from build123d import *

# Parameters (mm, degrees)
BOSS_EXTRUDE1_DEPTH  = 10
MIRROR1_DEPTH        = 10
SKETCH2_R            = 17.5
SKETCH2_R_2          = 15.5
BOSS_EXTRUDE2_DEPTH  = 5
CUT_EXTRUDE2_START   = -5
SKETCH3_R            = 15.5
CUT_EXTRUDE2_DEPTH   = 5
SKETCH4_R            = 12.5
CUT_EXTRUDE3_DEPTH   = 81.734131568
CHAMFER2_SIZE        = 0.2
CHAMFER4_SIZE        = 0.5
SKETCH5_R            = 5
SKETCH5_R_2          = 21
CUT_EXTRUDE5_DEPTH   = 1
CHAMFER6_SIZE        = 1
SKETCH6_R            = 0.75
CUT_EXTRUDE6_DEPTH   = 7
SKETCH7_R            = 0.75
CUT_EXTRUDE7_DEPTH   = 7
CUT_EXTRUDE8_DEPTH   = 151.432709209
CUT_EXTRUDE9_DEPTH   = 100.548982918
CUT_EXTRUDE10_DEPTH  = 81.616375508
FILLET3_R            = 2
FILLET3_OF_MIRROR3_R = 2
SKETCH11_R           = 0.75
CUT_EXTRUDE11_DEPTH  = 5


# Read off the part's stored shape, not the designer's step: Mirror1
with BuildPart() as part:
    # Sketch1 → Boss-Extrude1 (new body)
    with BuildSketch(Plane(origin=(0, 0, 0), x_dir=(1, 0, 0), z_dir=(0, 1, 0))):
        Polygon((-73, 31), (-71, 33), (-63, 33), (-61, 31), (-7, 31), (-5, 33), (0, 33), (0, 0), (-73, 0), (-73, 5), (-71, 7), (-71, 21), (-73, 23), align=None)
    extrude(amount=BOSS_EXTRUDE1_DEPTH)

    # Mirror1 outline → Mirror1 (add)
    with BuildSketch(Plane(origin=(0, 0, 0), x_dir=(1, 0, 0), z_dir=(0, 1, 0))):
        Polygon((-73, 0), (-73, -5), (-71, -7), (-71, -21), (-73, -23), (-73, -31), (-71, -33), (-63, -33), (-61, -31), (-7, -31), (-5, -33), (5, -33), (7, -31), (61, -31), (63, -33), (71, -33), (73, -31), (73, -23), (71, -21), (71, -7), (73, -5), (73, 5), (71, 7), (71, 21), (73, 23), (73, 31), (71, 33), (63, 33), (61, 31), (7, 31), (5, 33), (0, 33), (0, 0), align=None)
    extrude(amount=MIRROR1_DEPTH)

    # Sketch2 → Boss-Extrude2 (add)
    with BuildSketch(Plane(origin=(0, 10, 0), x_dir=(1, 0, 0), z_dir=(0, 1, 0))):
        with Locations(Location((0, 0, 0), (0, 0, 90))):
            Circle(SKETCH2_R)
        with Locations(Location((0, 0, 0), (0, 0, 270))):
            Circle(SKETCH2_R_2, mode=Mode.SUBTRACT)
    extrude(amount=BOSS_EXTRUDE2_DEPTH)

    # Sketch3 → Cut-Extrude2 (cut)
    with BuildSketch(Plane(origin=(0, 10, 0), x_dir=(1, 0, 0), z_dir=(0, 1, 0)).offset(CUT_EXTRUDE2_START)):
        with Locations(Location((0, 0, 0), (0, 0, 270))):
            Circle(SKETCH3_R)
    extrude(amount=CUT_EXTRUDE2_DEPTH, mode=Mode.SUBTRACT)

    # Sketch4 → Cut-Extrude3 (cut, through all)
    with BuildSketch(Plane(origin=(0, 5, 0), x_dir=(1, 0, 0), z_dir=(0, 1, 0))):
        with Locations(Location((0, 0, 0), (0, 0, 270))):
            Circle(SKETCH4_R)
    extrude(amount=-CUT_EXTRUDE3_DEPTH, mode=Mode.SUBTRACT)

    # Chamfer2
    chamfer2_edges = [part.edges().sort_by_distance(p)[0] for p in [
        (0, 15, 17.5),
        (0, 15, -15.5),
    ]]
    chamfer(chamfer2_edges, length=CHAMFER2_SIZE)

    # Chamfer4
    chamfer4_edges = [part.edges().sort_by_distance(p)[0] for p in [
        (0, 0, -12.5),
        (0, 5, -12.5),
    ]]
    chamfer(chamfer4_edges, length=CHAMFER4_SIZE)

    # Sketch5 → Cut-Extrude5 (cut)
    with BuildSketch(Plane.XZ.offset(-10)):
        Polygon((71, 4.171572875), (69, 6.171572875), (69, 21.828427125), (71, 23.828427125), (71, 30.171572875), (70.171572875, 31), (63.828427125, 31), (61.828427125, 29), (6.171572875, 29), (4.171572875, 31), (-4.171572875, 31), (-6.171572875, 29), (-61.828427125, 29), (-63.828427125, 31), (-70.171572875, 31), (-71, 30.171572875), (-71, 23.828427125), (-69, 21.828427125), (-69, 6.171572875), (-71, 4.171572875), (-71, -4.171572875), (-69, -6.171572875), (-69, -21.828427125), (-71, -23.828427125), (-71, -30.171572875), (-70.171572875, -31), (-63.828427125, -31), (-61.828427125, -29), (-6.171572875, -29), (-4.171572875, -31), (4.171572875, -31), (6.171572875, -29), (61.828427125, -29), (63.828427125, -31), (70.171572875, -31), (71, -30.171572875), (71, -23.828427125), (69, -21.828427125), (69, -6.171572875), (71, -4.171572875), align=None)
        with Locations(Location((-42.5, 0, 0), (0, 0, 270))):
            Circle(SKETCH5_R, mode=Mode.SUBTRACT)
        with Locations(Location((42.5, 0, 0), (0, 0, 270))):
            Circle(SKETCH5_R, mode=Mode.SUBTRACT)
        with Locations(Location((0, 0, 0), (0, 0, 270))):
            Circle(SKETCH5_R_2, mode=Mode.SUBTRACT)
    extrude(amount=CUT_EXTRUDE5_DEPTH, mode=Mode.SUBTRACT)

    # Chamfer6
    chamfer6_edges = [part.edges().sort_by_distance(p)[0] for p in [
        (0, 9, 21),
        (67, 9, 31),
        (62.828427125, 9, 30),
        (34, 9, 29),
        (5.171572875, 9, 30),
        (0, 9, 31),
        (-5.171572875, 9, 30),
        (-34, 9, 29),
        (-62.828427125, 9, 30),
        (-67, 9, 31),
        (-71, 9, 27),
        (-70, 9, 22.828427125),
        (-69, 9, 14),
        (-70, 9, 5.171572875),
        (-71, 9, 0),
        (-70, 9, -5.171572875),
        (-69, 9, -14),
        (-70, 9, -22.828427125),
        (-71, 9, -27),
        (-67, 9, -31),
        (-62.828427125, 9, -30),
        (-34, 9, -29),
        (-5.171572875, 9, -30),
        (0, 9, -31),
        (5.171572875, 9, -30),
        (34, 9, -29),
        (62.828427125, 9, -30),
        (67, 9, -31),
        (71, 9, -27),
        (70, 9, -22.828427125),
        (69, 9, -14),
        (70, 9, -5.171572875),
        (71, 9, 0),
        (70, 9, 5.171572875),
        (69, 9, 14),
        (70, 9, 22.828427125),
        (71, 9, 27),
        (70.585786438, 9, 30.585786438),
        (-70.585786438, 9, 30.585786438),
        (-70.585786438, 9, -30.585786438),
        (70.585786438, 9, -30.585786438),
        (-42.5, 9, 5),
        (42.5, 9, 5),
    ]]
    chamfer(chamfer6_edges, length=CHAMFER6_SIZE - 0.0001)  # a hair under: the kernel refuses the full size

    # Sketch6 → Cut-Extrude6 (cut)
    with BuildSketch(Plane.XY.offset(33)):
        with Locations((0, 5)):
            Circle(SKETCH6_R)
    cut_extrude6 = extrude(amount=-CUT_EXTRUDE6_DEPTH, mode=Mode.SUBTRACT)

    # Mirror2: Cut-Extrude6 across plane
    add(cut_extrude6.mirror(Plane.XY), mode=Mode.SUBTRACT)

    # Sketch7 → Cut-Extrude7 (cut)
    with BuildSketch(Plane(origin=(0, 10, 0), x_dir=(1, 0, 0), z_dir=(0, 1, 0))):
        with Locations(Location((-42.5, 0, 0), (0, 0, 270))):
            Circle(SKETCH7_R)
        with Locations(Location((42.5, 0, 0), (0, 0, 270))):
            Circle(SKETCH7_R)
    extrude(amount=-CUT_EXTRUDE7_DEPTH, mode=Mode.SUBTRACT)

    # Sketch8 → Cut-Extrude8 (cut, through all)
    with BuildSketch(Plane.ZY.offset(73)):
        Polygon((-33, 9), (-32, 10), (-33, 10), align=None)
        Polygon((33, 10), (32, 10), (33, 9), align=None)
    extrude(amount=-CUT_EXTRUDE8_DEPTH, mode=Mode.SUBTRACT)

    # Sketch9 → Cut-Extrude9 (cut, through all)
    with BuildSketch(Plane.XY.offset(33)):
        Polygon((-73, 10), (-72, 10), (-73, 9), align=None)
        Polygon((72, 10), (73, 10), (73, 9), align=None)
    extrude(amount=-CUT_EXTRUDE9_DEPTH, mode=Mode.SUBTRACT)

    # Sketch10 → Cut-Extrude10 (cut, through all)
    with BuildSketch(Plane(origin=(0, 9, 0), x_dir=(1, 0, 0), z_dir=(0, 1, 0))):
        with BuildLine():
            ThreePointArc((-19.342622189, 16.230387145), (-19.835649522, 21.865715356), (-25.470977734, 21.372688022))
            ThreePointArc((-25.470977734, 21.372688022), (-33.25, 0), (-25.470977734, -21.372688022))
            ThreePointArc((-25.470977734, -21.372688022), (-19.835649522, -21.865715356), (-19.342622189, -16.230387145))
            ThreePointArc((-19.342622189, -16.230387145), (-25.25, 0), (-19.342622189, 16.230387145))
        make_face()
    cut_extrude10 = extrude(amount=-CUT_EXTRUDE10_DEPTH, mode=Mode.SUBTRACT)

    # Fillet3
    fillet3_edges = [part.edges().sort_by_distance(p)[0] for p in [
        (-33.25, 0, 0),
        (-19.835649522, 0, -21.865715356),
        (-25.25, 0, 0),
        (-19.835649522, 0, 21.865715356),
    ]]
    fillet(fillet3_edges, radius=FILLET3_R)

    # Mirror3: Cut-Extrude10 across plane
    add(cut_extrude10.mirror(Plane(origin=(0, 0, 0), x_dir=(0, 0, 1), z_dir=(1, 0, 0))), mode=Mode.SUBTRACT)

    # Fillet3 of Mirror3
    fillet3_of_mirror3_edges = [part.edges().sort_by_distance(p)[0] for p in [
        (33.25, 0, 0),
        (19.835649522, 0, -21.865715356),
        (25.25, 0, 0),
        (19.835649522, 0, 21.865715356),
    ]]
    fillet(fillet3_of_mirror3_edges, radius=FILLET3_OF_MIRROR3_R)

    # Sketch11 → Cut-Extrude11 (cut)
    with BuildSketch(Plane.XZ):
        with Locations(Location((0, 17.2, 0), (0, 0, 270))):
            Circle(SKETCH11_R)
        with Locations(Location((45.6, 10.2, 0), (0, 0, 270))):
            Circle(SKETCH11_R)
        with Locations(Location((45.6, -10.2, 0), (0, 0, 270))):
            Circle(SKETCH11_R)
        with Locations(Location((0, -17.2, 0), (0, 0, 270))):
            Circle(SKETCH11_R)
    extrude(amount=-CUT_EXTRUDE11_DEPTH, mode=Mode.SUBTRACT)


solid = part.part
Can you work these out from the model? Positions are in its coordinate system, mm. A direction names the side the tool comes from. Coordinates: 2 decimals unless noted, no trailing zeros. Return JSON: item names as keys, results as strings. Group by question number.
Item 1: On a 3-axis mill with a long thin cutter (end or side, diameter ignored), from which of +Z, -Z, +X, -X, +Y, -Y can I reach the whole of each face in a straight line? I mean faces 1 (the flat face through (-34, 5, -31)), 2 (the flat face through (71, 5, 14)), 3 (the flat face through (44, 10, 0)), 4 (the flat face through (-69.479, 9.493, -23.024)), 5 (the cylindrical face through (25.25, 5.55, 0.25)). Say none if no direction works.
Item 2: If I drill on L1, parallel to Z at x = 45.6, y = 2.75; L2, parallel to X at y = 1.8, z = -10.2; L3, parallel to Z at x = -42.5, y = 5, over which ranges is the centre line in solid material (lowest first)? Write a range as from..to.
Item 3: I'm going to push flat-ended pins straight in: pin 1 Ø8 at (x, y) = (40, 6) entering from -Z; pin 2 Ø6 at (x, y) = (-52.5, 12) entering from +Z; pin 3 Ø12 at (x, z) = (-20.5, 21) entering from -Y; pin 4 Ø11 at (x, z) = (-42.5, -1.5) entering from +Y. Where does each tip first touch, or does it pass through?
Item 4: Thinking about a two-plate mould opening in Z: for faces 6 (the flat face through (-13, 5, 3)), 7 (the cylindrical face through (10.648, 12.366, 13.887)), 8 (the flat face through (-8, 10, -16)), 9 (the flat face through (34, 5, 31)), which applies, released by +Z, released by -Z, zero draft, split by the parting line, or undercut?
Verdict:
{
 "1": {"face 1": "-Z, +Y, -Y", "face 2": "+X, +Y, -Y", "face 3": "+Z, -Z, +X, +Y", "face 4": "+Y", "face 5": "+Y, -Y"},
 "2": {"L1": "z = -31..-10.95, -9.45..9.45, 10.95..31", "L2": "x = -71..-31.66, -23.09..-7.23, 7.23..23.09, 31.66..44.85, 46.35..71", "L3": "z = -31..-0.75, 0.75..31"},
 "3": {"pin 1": "stops at z = -31", "pin 2": "stops at z = 31", "pin 3": "stops at y = 0", "pin 4": "stops at y = 10"},
 "4": {"face 6": "undercut", "face 7": "split by the parting line", "face 8": "zero draft", "face 9": "released by +Z"}
}
